Can you work these out from the drawing? Everything is in mm from the part's minimum corner. A direction names the side the tool comes from. Round coordinates to 2 decimals unless told otherwise and drop trailing zeros. Loops run counter-clockwise (first coordinate to the right, second up) from the corner with the lowest first, then second, coordinate; pieces in that order, holes last. Notation, with made-up numbers: (11, -31) - (48, -31) arc R24 cw to (48, -6) - close; hole circle Ø6 at (30.25, -18). An arc over 180 degrees is marked (long way). Return JSON: item names as keys, results as strings. Group by question number.
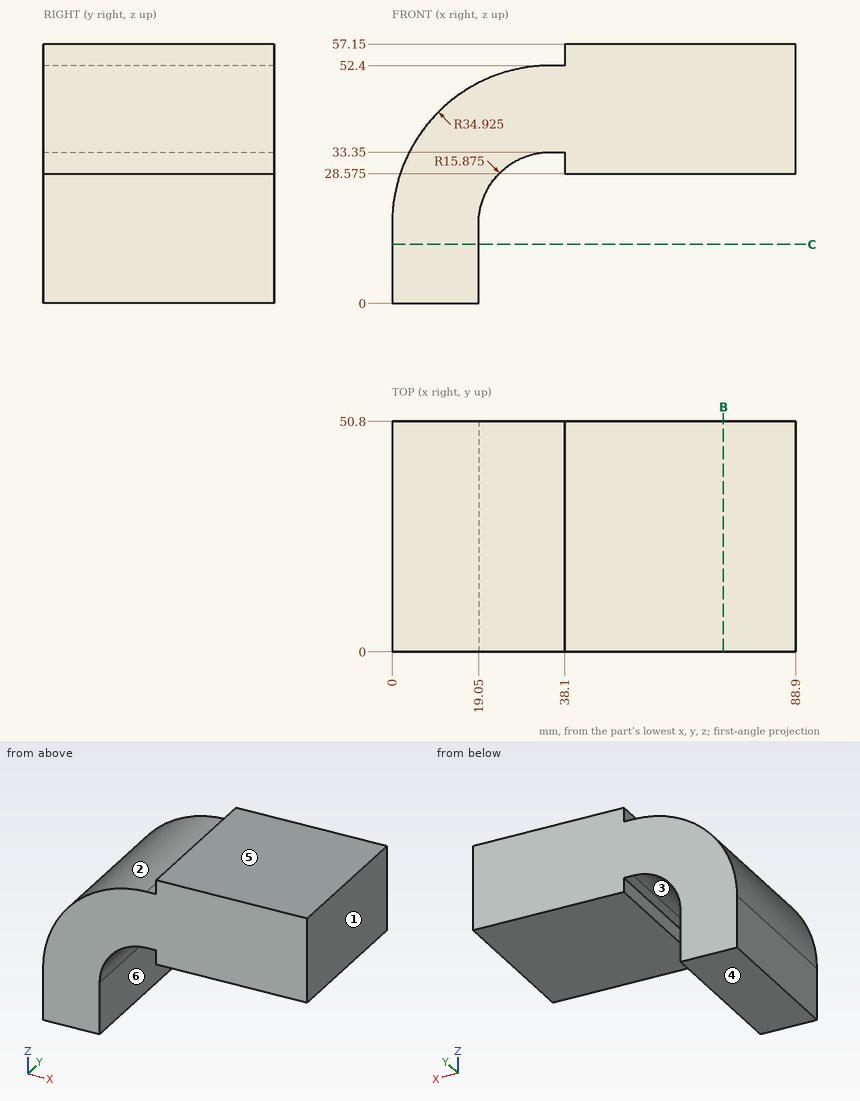
Q1. For the marked faces 5 and 6, which set-ups out of +Z, -Z, +X, -X, +Y, -Y let a thin tool reach every point of the face, with its end or its side?
Q2. Imagine slicing it at C-C, the plane z = 13. List the corners of the cut face in (x, y) for me.
Q3. Imagine slicing it at B-B, the plane x = 73. List the corners of the cut face in (y, z) for me (3 decimals).
Q4. If we mould it in two halves opening along X, with no side actions, what happens to the marked faces 1, 2, 3 and 4? For each: +X half, -X half, draft (parallel to the pull), parting line (faces both ways), or undercut.
Q5. Will these pins go through, and if not, where does the flat tip stop? pin 1 Ø2 at (x, y) = (26.5, 15) entering from -Z; pin 2 Ø3 at (y, z) = (37.5, 30.5) entering from -X; pin 3 Ø2 at (x, y) = (61, 18) entering from -Z (3 decimals).
Q6. Please list where these lines run through material, in increasing order: line 1 (X direction, y = 13, z = 54); line 2 (Z direction, x = 45.5, y = 6) (3 decimals); line 3 (X direction, y = 29, z = 29).
Output values:
{
 "1": {"face 5": "+Z, +X, -X, +Y, -Y", "face 6": "-Z, +X, +Y, -Y"},
 "2": {"outline": "(0, 0) - (19.05, 0) - (19.05, 50.8) - (0, 50.8) - close"},
 "3": {"outline": "(0, 28.575) - (50.8, 28.575) - (50.8, 57.15) - (0, 57.15) - close"},
 "4": {"face 1": "+X half", "face 2": "-X half", "face 3": "undercut", "face 4": "draft"},
 "5": {"pin 1": "stops at z = 30.25", "pin 2": "stops at x = 1.96", "pin 3": "stops at z = 28.575"},
 "6": {"line 1": "x = 38.1 to 88.9", "line 2": "z = 28.575 to 57.15", "line 3": "x = 1.96 to 24.01, 38.1 to 88.9"}
}
